from build123d import *

# Parameters (mm, degrees)
SKETCH3_R               = 1.25
BOSS_EXTRUDE2_DEPTH     = 36
CUT_EXTRUDE1_DEPTH      = 53.24200467
CUT_EXTRUDE1_DEPTH_BACK = 53.24200467
SKETCH4_W               = 13.5
SKETCH4_H               = 5
BOSS_EXTRUDE3_DEPTH     = 30


with BuildPart() as part:
    # Sketch3 → Boss-Extrude2 (new, symmetric)
    with BuildSketch(Plane(origin=(0, 0, 0), x_dir=(0, 0, -1), z_dir=(1, 0, 0))):
        with BuildLine():
            Line((-35.75, 2.857368006), (35.75, 2.857368006))
            Line((35.75, 2.857368006), (35.75, -1.142631994))
            Line((35.75, -1.142631994), (-35.75, -1.142631994))
            ThreePointArc((-35.75, -1.142631994), (-37.75, 0.857368006), (-35.75, 2.857368006))
        make_face()
        with Locations((-35.75, 0.857368006)):
            Circle(SKETCH3_R, mode=Mode.SUBTRACT)
    extrude(amount=BOSS_EXTRUDE2_DEPTH, both=True)

    # Sketch4 → Cut-Extrude1 (cut, two sides: drawn at the far end of the back side and taken through both)
    with BuildSketch(Plane(origin=(0, 0, 0), x_dir=(1, 0, 0), z_dir=(0, 1, 0)).offset(-CUT_EXTRUDE1_DEPTH_BACK)):
        with Locations((-29.25, -35.25)):
            Rectangle(SKETCH4_W, SKETCH4_H)
        with Locations((29.25, -35.25)):
            Rectangle(SKETCH4_W, SKETCH4_H)
        with Locations((0, -35.25)):
            Rectangle(SKETCH4_W, SKETCH4_H)
    extrude(amount=CUT_EXTRUDE1_DEPTH + CUT_EXTRUDE1_DEPTH_BACK, mode=Mode.SUBTRACT)

    # Sketch7 → Boss-Extrude3 (add, symmetric)
    with BuildSketch(Plane(origin=(0, 0, 0), x_dir=(0, 0, -1), z_dir=(1, 0, 0))):
        Polygon((30.876330293, -1.142631994), (30.876330293, -3.878672559), (19.808295325, -1.142631994), align=None)
    extrude(amount=BOSS_EXTRUDE3_DEPTH, both=True)


solid = part.part
CAD build for the part. Positions are in the model's coordinates, mm. A direction names the side the tool comes from. Round coordinates to 2 decimals unless told otherwise and drop trailing zeros. Loops run counter-clockwise (first coordinate to the right, second up) from the corner with the lowest first, then second, coordinate; pieces in that order, holes last. Notation, with made-up numbers: (43.25, -10.75) - (78.25, -10.75) arc R29 cw to (78.25, 27.25) - close; hole circle Ø6 at (56.5, 37). An arc over 180 degrees is marked (long way). Put each result on its own line as item: value.
1. 3-axis set-ups, long thin cutter, end or side, ignore diameter. For faces 1 (the flat face through (-22.5, 1, 34)), 2 (the flat face through (0, 1, 32.75)), 3 (the flat face through (29, 1, 32.75)), 4 (the flat face through (-30, -2, -27)), 5 (the flat face through (0, -2, -30.876)): which of +Z, -Z, +X, -X, +Y, -Y reach the whole face in a straight line?
Geometry check:
face 1: +Z, -X, +Y, -Y
face 2: +Z, +Y, -Y
face 3: +Z, +X, +Y, -Y
face 4: +Z, -Z, -X, -Y
face 5: -Z, +X, -X, -Y
2. Pin check, flat tips, straight feed: P1, Ø2, axis at y = 0.86, z = 35.75, coming from the +X side; P2, Ø10, axis at x = -7.5, z = 3, coming from the -Y side; P3, Ø4, axis at y = 0.86, z = 35.75, coming from the -X side; P4, Ø1.2, axis at y = 0, z = 35.5, coming from the +X side. Stop position of each tip, or through.
Geometry check:
P1: through
P2: y = -1.14
P3: x = -22.5
P4: x = 22.5
3. Slice it at A-A on x = -23.5. List the corners of the cut face in (y, z), and give its area (3 significant figures).
Geometry check:
outline: (-3.88, -30.88) - (-1.14, -30.88) - (-1.14, -35.75) - (2.86, -35.75) - (2.86, 32.75) - (-1.14, 32.75) - (-1.14, -19.81) - close
area: 289 mm²
4. Slice it at B-B on x = -10. List the corners of the cut face in (y, z), and give its area (3 significant figures).
Geometry check:
outline: (-3.88, -30.88) - (-1.14, -30.88) - (-1.14, -35.75) - (2.86, -35.75) - (2.86, 35.75) arc R2 ccw to (-1.14, 35.75) - (-1.14, -19.81) - close; hole circle Ø2.5 at (0.86, 35.75)
area: 303 mm²
5. Two-plate mould, pull along X, no slides. Class faces 6 (the flat face through (-6.75, 1, 34)), 7 (the flat face through (-29, 1, 32.75)), 8 (the flat face through (6.75, 1, 34)), 9 (the flat face through (30, -2, -27)): released by +X, released by -X, zero draft, split by the parting line, or undercut.
Geometry check:
face 6: undercut
face 7: zero draft
face 8: undercut
face 9: released by +X
6. Slice it at C-C on z = -28. List the corners of the cut face in (x, y), and give its area (4 significant figures).
Geometry check:
outline: (-36, -1.14) - (-30, -1.14) - (-30, -3.17) - (30, -3.17) - (30, -1.14) - (36, -1.14) - (36, 2.86) - (-36, 2.86) - close
area: 409.5 mm²
7. Slice it at D-D on z = -1. List the corners of the cut face in (x, y).
Geometry check:
outline: (-36, -1.14) - (36, -1.14) - (36, 2.86) - (-36, 2.86) - close
8. Wall check: line 1 (Y direction, x = 10.75, z = 35.75); line 2 (Y direction, x = -7, z = 19); line 3 (Z direction, x = 1.5, y = 1). Give the ranges that are in metal, low to high.
Geometry check:
line 1: -1.14 to -0.39, 2.11 to 2.86
line 2: -1.14 to 2.86
line 3: -35.75 to 32.75
